from build123d import *

# Parameters (mm, degrees)
F0_R     = 3.81
F1_DEPTH = 12.7
F2_DEPTH = 12.7
F3_T     = -7.62
F5_DEPTH = 10.16


with BuildPart() as f1:
    # F0 (on Top) → F1 (new body)
    with BuildSketch(Plane.XY):
        with BuildLine():
            ThreePointArc((13.0135805012, 21.8129943506), (-22.0873826509, -12.5422297712), (25.4, 0))
            ThreePointArc((25.4, 0), (23.5709280626, 9.4642141917), (18.3471377744, 17.5653788883))
            ThreePointArc((18.3471377744, 17.5653788883), (7.7542007796, 9.7366332552), (13.0135805012, 21.8129943506))
        make_face()
        Circle(F0_R, mode=Mode.SUBTRACT)
        with BuildLine():
            ThreePointArc((13.0135805012, 21.8129943506), (7.7542007796, 9.7366332552), (18.3471377744, 17.5653788883))
            ThreePointArc((18.3471377744, 17.5653788883), (15.8235338016, 19.8689651978), (13.0135805012, 21.8129943506))
        make_face()
    extrude(amount=F1_DEPTH)

    # F2 (add): a face of the model
    f2_faces = [f1.faces().sort_by_distance(p)[0] for p in [
        (-24.6815795103, 0, 12.7),
    ]]
    extrude(f2_faces, amount=F2_DEPTH)

    # F3
    f3_openings = [f1.faces().sort_by_distance(p)[0] for p in [
        (-25.4, 0, 12.7),
    ]]
    offset(amount=F3_T, openings=f3_openings)

    # F4 (on face) → F5 (cut)
    with BuildSketch(Plane.XY.offset(25.4)):
        with BuildLine():
            ThreePointArc((22.3176650745, 12.1277296154), (20.5505059881, 14.927715955), (18.434145823, 17.4740455469))
            ThreePointArc((18.434145823, 17.4740455469), (12.1795633167, 8.8471330951), (22.3176650745, 12.1277296154))
        make_face()
    extrude(amount=-F5_DEPTH, mode=Mode.SUBTRACT)


solid = f1.part
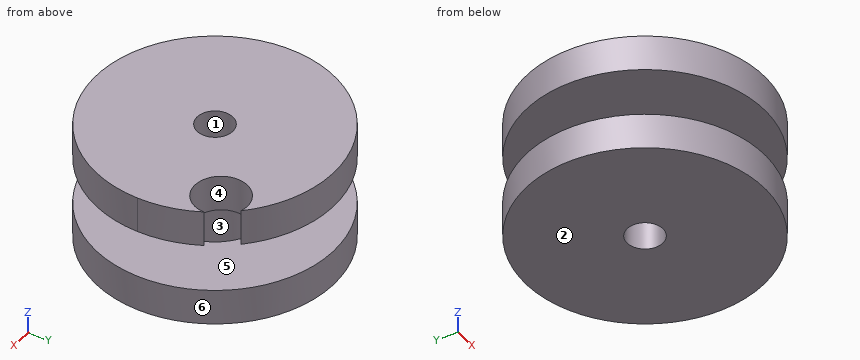
Can you work these out from the model? Positions are in its coordinate system, mm. Face numbers are marked on the shaded views. A direction names the side the tool comes from. Give positions to 0.01 mm unless a question says otherwise; leave off trailing zeros. Loops run counter-clockwise (first coordinate to the right, second up) from the corner with the lowest first, then second, coordinate; pieces in that order, holes last. Notation, with made-up numbers: (82, 23) -> (133, 23) arc R32 ccw to (133, 55) -> close; hole circle Ø3 at (-14, 65.25). An arc over 180 degrees is marked (long way). Return JSON: item names as keys, results as strings.
Q1. We'd pull the mould along Z, two halves only. Please class the marked faces 1, 2 and 3: released by +Z, released by -Z, zero draft, split by the parting line, or undercut.
Checks:
{"face 1": "zero draft", "face 2": "released by -Z", "face 3": "undercut"}
Q2. I need wall thicknesses on probe 1 along Z at (x, y) = (11, 4); probe 2 along Y at (x, z) = (0, 6.75); probe 3 along Y at (x, z) = (1, 2.25). Which ranges of each line are inside material? Lowest first, please.
Checks:
{"probe 1": "z = 0 to 7.62, 17.78 to 25.4", "probe 2": "y = -25.4 to -3.81, 3.81 to 25.4", "probe 3": "y = -25.38 to -3.68, 3.68 to 25.38"}
Q3. I want a section at D-D, the plane x = -19.5. List the corners of the cut face in (y, z) for me.
Checks:
{"outline": "(-16.28, 0) -> (16.28, 0) -> (16.28, 7.62) -> (-16.28, 7.62) -> close; (-16.28, 17.78) -> (16.28, 17.78) -> (16.28, 25.4) -> (-16.28, 25.4) -> close"}
Q4. I want a section at C-C, the plane y = 7.5. List the corners of the cut face in (x, z) for me.
Checks:
{"outline": "(-24.27, 0) -> (24.27, 0) -> (24.27, 7.62) -> (8.63, 7.62) -> (8.63, 17.78) -> (13.57, 17.78) -> (13.57, 25.4) -> (-24.27, 25.4) -> (-24.27, 17.78) -> (-8.63, 17.78) -> (-8.63, 7.62) -> (-24.27, 7.62) -> close; (19.86, 17.78) -> (24.27, 17.78) -> (24.27, 25.4) -> (19.86, 25.4) -> close"}
Q5. I want a section at A-A, the plane x = 0. List the corners of the cut face in (y, z) for me, then the cut area to 3 significant figures.
Checks:
{"outline": "(-25.4, 0) -> (-3.81, 0) -> (-3.81, 25.4) -> (-25.4, 25.4) -> (-25.4, 17.78) -> (-11.43, 17.78) -> (-11.43, 7.62) -> (-25.4, 7.62) -> close; (3.81, 0) -> (25.4, 0) -> (25.4, 7.62) -> (11.43, 7.62) -> (11.43, 17.78) -> (25.4, 17.78) -> (25.4, 25.4) -> (3.81, 25.4) -> close", "area": "813 mm2"}
Q6. For pin 1 Ø13 at (x, y) = (16.71, 12.14) entering from +Z; pin 2 Ø12 at (y, z) = (9, 16) entering from +X; pin 3 Ø2 at (x, z) = (-4, 7) entering from -Y; pin 4 Ø1 at (y, z) = (-12.5, 23) entering from +X, each with a flat end and sliding along its axis, tell me the tip position at first contact or that it passes through.
Checks:
{"pin 1": "stops at z = 25.4", "pin 2": "stops at x = 25.19", "pin 3": "stops at y = -25.22", "pin 4": "stops at x = 22.39"}
Q7. On a 3-axis mill with a long thin cutter (end or side, diameter ignored), from which of +Z, -Z, +X, -X, +Y, -Y can I reach the whole of each face in a straight line? I mean the marked faces 4, 5 and 6. Say none if no direction works.
Checks:
{"face 4": "+Z", "face 5": "none", "face 6": "+Z, -Z"}
Q8. I want a section at B-B, the plane z = 6. List the corners of the cut face in (x, y) for me, then the cut area to 3 significant figures.
Checks:
{"outline": "circle Ø50.8 at (0, 0); hole circle Ø7.62 at (0, 0)", "area": "1,980 mm2"}
